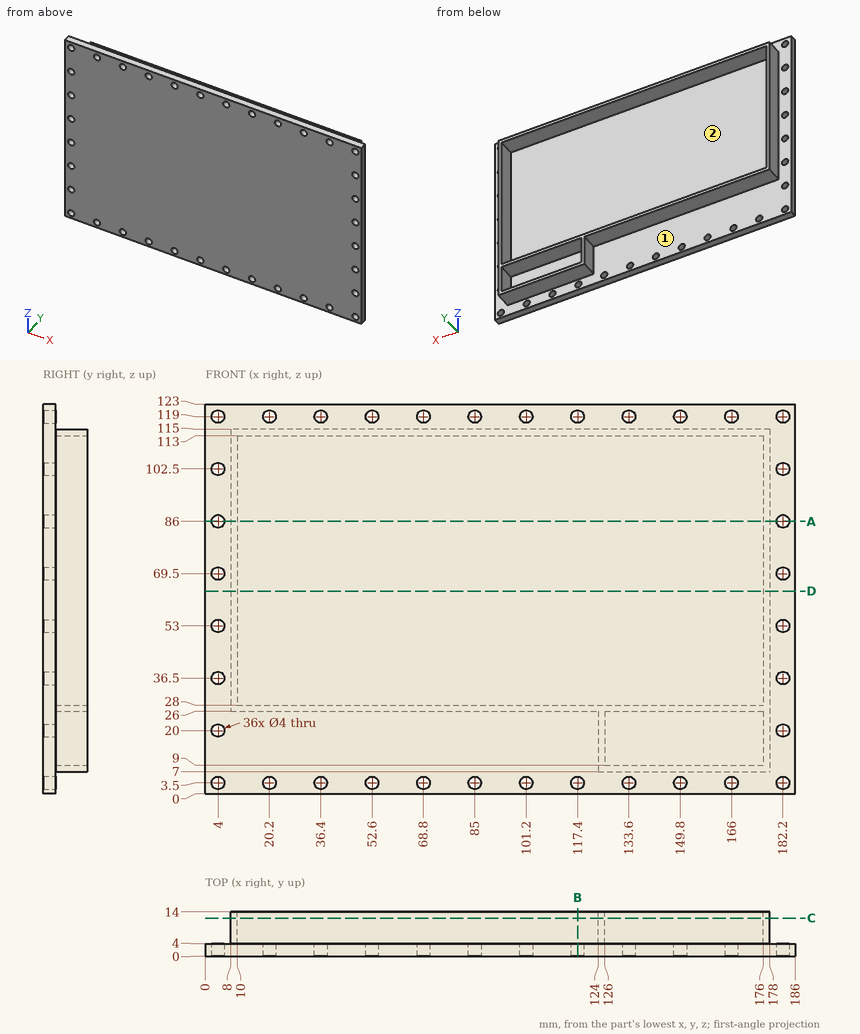
For this review, use the dimensioned drawing (mm, ordinates from the lowest corner) and the shaded views. Round coordinates to 2 decimals unless told otherwise and drop trailing zeros. Order: outer loops, then holes, each group sorted by start corner. A loop starts at its lowest first (then second) coordinate and runs counter-clockwise, first axis right, second up. Notation, with made-up numbers: M 22.5,60.5 L 33.5,60.5 A17 cw 33.5,72.5 Z; hole C -3.5,11.5 d2. An arc over 180 degrees is marked long. Use a Markdown table: item, result. Add a question column.
Item 1: Add section C-C, the plane y = 12. Give the boundary of the cut face in (x, z), then the cut area to 3 significant figures.
Item 2: Insertion check: pin 1 (3 mm diameter, centred on x = 58.5, y = 7.5, fed in from -Z); pin 2 (8 mm diameter, centred on x = 121.5, z = 51.5, fed in from +Y); pin 3 (3 mm diameter, centred on x = 124, y = 12, fed in from +Z). Each pin has a flat end and moves straight along its axis. Give the tip position at first contact, or say it passes through.
Item 3: Mouldability with a two-part tool opening along Z and no side actions: class the marked faces 1 and 2 as released by +Z, released by -Z, zero draft, split by the parting line, or undercut.
Item 4: Add section A-A, the plane z = 86. Give the boundary of the cut face in (x, y), then the cut area to 3 significant figures.
Item 5: Add section D-D, the plane z = 64. Give the boundary of the cut face in (x, y), then the cut area to 3 significant figures.
Item 6: Add section B-B, the plane x = 117.4. Give the boundary of the cut face in (y, z).
Item 7: To check wall thickness, follow line 1 along X through (y, z) = (1.5, 20); line 2 along Z through (x, y) = (85, 2.2); line 3 along Z through (x, y) = (127, 12.25). State the ranges of each line that lie inside material, in increasing order.
Geometry results:
| question | item | result |
|---|---|---|
| 1 | outline | M 8,26 L 124,26 L 124,7 L 178,7 L 178,115 L 8,115 Z; hole M 10,28 L 176,28 L 176,113 L 10,113 Z; hole M 126,9 L 176,9 L 176,26 L 126,26 Z |
| 1 | area | 1,200 mm² |
| 2 | pin 1 | stops at z = 26 |
| 2 | pin 2 | stops at y = 4 |
| 2 | pin 3 | stops at z = 115 |
| 3 | face 1 | zero draft |
| 3 | face 2 | undercut |
| 4 | outline | M 0,0 L 2,0 L 2,4 L 0,4 Z; M 6,0 L 180.2,0 L 180.2,4 L 178,4 L 178,14 L 176,14 L 176,4 L 10,4 L 10,14 L 8,14 L 8,4 L 6,4 Z; M 184.2,0 L 186,0 L 186,4 L 184.2,4 Z |
| 4 | area | 752 mm² |
| 5 | outline | M 0,0 L 186,0 L 186,4 L 178,4 L 178,14 L 176,14 L 176,4 L 10,4 L 10,14 L 8,14 L 8,4 L 0,4 Z |
| 5 | area | 784 mm² |
| 6 | outline | M 0,0 L 4,0 L 4,1.5 L 0,1.5 Z; M 0,5.5 L 4,5.5 L 4,26 L 14,26 L 14,28 L 4,28 L 4,113 L 14,113 L 14,115 L 4,115 L 4,117 L 0,117 Z; M 0,121 L 4,121 L 4,123 L 0,123 Z |
| 7 | line 1 | x = 0 to 2, 6 to 180.2, 184.2 to 186 |
| 7 | line 2 | z = 0 to 1.5, 5.5 to 117, 121 to 123 |
| 7 | line 3 | z = 7 to 9, 26 to 28, 113 to 115 |
